Design review of the part built by this model. Coordinates are the model's own, in mm. Coordinates: 2 decimals unless noted, no trailing zeros. Order: outer loops, then holes, each group sorted by start corner. A loop starts at its lowest first (then second) coordinate and runs counter-clockwise, first axis right, second up.
from build123d import *

# Parameters (mm, degrees)
SKETCH2_W           = 10
SKETCH2_H           = 60
SKETCH2_R           = 2.5
BOSS_EXTRUDE1_DEPTH = 4
FILLET1_R           = 1


with BuildPart() as part:
    # Sketch2 → Boss-Extrude1 (new body)
    with BuildSketch(Plane.XY):
        with Locations((5, 30)):
            Rectangle(SKETCH2_W, SKETCH2_H)
        with Locations((5, 50)):
            Circle(SKETCH2_R, mode=Mode.SUBTRACT)
        with Locations((5, 10)):
            Circle(SKETCH2_R, mode=Mode.SUBTRACT)
        with Locations((5, 30)):
            Circle(SKETCH2_R, mode=Mode.SUBTRACT)
    extrude(amount=BOSS_EXTRUDE1_DEPTH)

    # Fillet1
    fillet1_edges = [part.edges().sort_by_distance(p)[0] for p in [
        (10, 30, 4),
        (5, 60, 4),
        (0, 30, 4),
        (5, 60, 0),
        (10, 30, 0),
        (5, 0, 0),
        (0, 30, 0),
        (0, 60, 2),
        (10, 60, 2),
        (10, 0, 2),
        (0, 0, 2),
        (5, 0, 4),
    ]]
    fillet(fillet1_edges, radius=FILLET1_R)


solid = part.part
1. Add section D-D (y = 35). Give the boundary of the cut face in (x, z), and give its area (3 significant figures).
2. Add section A-A (y = 11.5). Give the boundary of the cut face in (x, z), and give its area (3 significant figures).
3. Add section C-C (z = 2). Give the boundary of the cut face in (x, y).
4. Mouldability with a two-part tool opening along X and no side actions: class faces 1 (the cylindrical face through (9.699, 0.285, 2.014)), 2 (the flat face through (8, 30, 4)), 3 (the cylindrical face through (7.385, 50.751, 1.972)) as pulls with the +X half, pulls with the -X half, needs draft (parallel to the pull), parting line crosses it, or undercut.
5. To check wall thickness, follow line 1 (Y direction, x = 5, z = 2); line 2 (Y direction, x = 2.75, z = 0.9); line 3 (X direction, y = 33, z = 3.5). State the ranges of each line that lie inside material, in increasing order.
6. Add section B-B (x = 5). Give the boundary of the cut face in (y, z).
7. Insertion check: pin 1 (1.5 mm diameter, centred on x = 3.5, y = 35.5, fed in from -Z); pin 2 (3 mm diameter, centred on x = 5, y = 10, fed in from -Z). Each pin has a flat end and moves straight along its axis. Give the tip position at first contact, or say it passes through.
Solution:
1. outline: (0, 1) arc R1 ccw to (1, 0) - (9, 0) arc R1 ccw to (10, 1) - (10, 3) arc R1 ccw to (9, 4) - (1, 4) arc R1 ccw to (0, 3) - close
1. area: 39.1 mm2
2. outline: (0, 1) arc R1 ccw to (1, 0) - (3, 0) - (3, 4) - (1, 4) arc R1 ccw to (0, 3) - close; (7, 0) - (9, 0) arc R1 ccw to (10, 1) - (10, 3) arc R1 ccw to (9, 4) - (7, 4) - close
2. area: 23.1 mm2
3. outline: (0, 1) arc R1 ccw to (1, 0) - (9, 0) arc R1 ccw to (10, 1) - (10, 59) arc R1 ccw to (9, 60) - (1, 60) arc R1 ccw to (0, 59) - close; hole circle Ø5 at (5, 10); hole circle Ø5 at (5, 30); hole circle Ø5 at (5, 50)
4. face 1: pulls with the +X half
4. face 2: needs draft
4. face 3: undercut
5. line 1: y = 0 to 7.5, 12.5 to 27.5, 32.5 to 47.5, 52.5 to 60
5. line 2: y = 0.01 to 8.91, 11.09 to 28.91, 31.09 to 48.91, 51.09 to 59.99
5. line 3: x = 0.13 to 9.87
6. outline: (0, 1) arc R1 ccw to (1, 0) - (7.5, 0) - (7.5, 4) - (1, 4) arc R1 ccw to (0, 3) - close; (12.5, 0) - (27.5, 0) - (27.5, 4) - (12.5, 4) - close; (32.5, 0) - (47.5, 0) - (47.5, 4) - (32.5, 4) - close; (52.5, 0) - (59, 0) arc R1 ccw to (60, 1) - (60, 3) arc R1 ccw to (59, 4) - (52.5, 4) - close
7. pin 1: stops at z = 0
7. pin 2: passes through
